Source: CAD feature listing. Evaluate the final solid. Frame: model axes, mm. Give positions to 0.01 mm unless a question says otherwise; leave off trailing zeros. Loops run counter-clockwise (first coordinate to the right, second up) from the corner with the lowest first, then second, coordinate; pieces in that order, holes last. Notation, with made-up numbers: (-6, 28) -> (37, 28) arc R18 cw to (37, 63) -> close; hole circle Ø5 at (24.25, 20). An arc over 180 degrees is marked (long way). Answer as a JSON object with one key per item and string values. Group by question number.
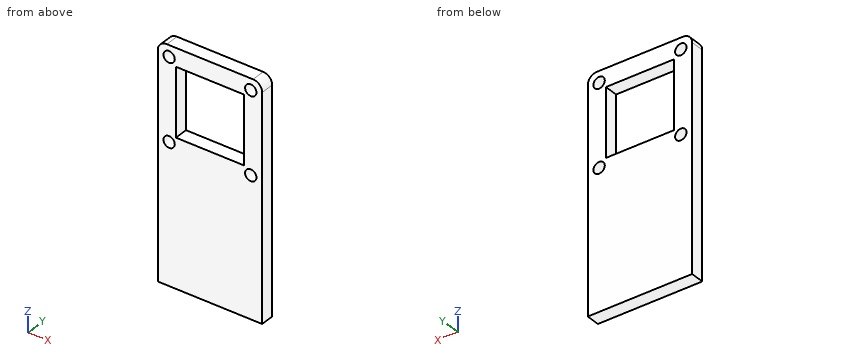
from build123d import *

# Parameters (mm, degrees)
F0_R     = 2.5
F0_W     = 30
F0_H     = 30
F1_DEPTH = 6


with BuildPart() as f1:
    # F0 (on Front) → F1 (new body)
    with BuildSketch(Plane.XZ):
        with BuildLine():
            ThreePointArc((23, 47), (21.828427, 49.828427), (19, 51))
            Line((19, 51), (-19, 51))
            ThreePointArc((-19, 51), (-21.828427, 49.828427), (-23, 47))
            Line((-23, 47), (-23, -51))
            Line((-23, -51), (23, -51))
            Line((23, -51), (23, 47))
        make_face()
        with Locations((-18, 10)):
            Circle(F0_R, mode=Mode.SUBTRACT)
        with Locations((-18, 46)):
            Circle(F0_R, mode=Mode.SUBTRACT)
        with Locations((18, 10)):
            Circle(F0_R, mode=Mode.SUBTRACT)
        with Locations((0, 28)):
            Rectangle(F0_W, F0_H, mode=Mode.SUBTRACT)
        with Locations((18, 46)):
            Circle(F0_R, mode=Mode.SUBTRACT)
    extrude(amount=F1_DEPTH)


solid = f1.part
(1) First-contact query: pin 1 (4 mm diameter, centred on x = -18, z = 10, fed in from -Y). Flat tip, straight axial feed; report the tip coordinate or a pass-through.
(2) Section query C-C on z = 10. Return the cut outline in (x, y), plus the area to 3 significant figures.
(3) Section query B-B on y = -3.05. Return the cut outline in (x, z), plus the area to 3 significant figures.
(4) Section query A-A on x = -7. Return the cut outline in (y, z).
(5) Section query D-D on x = -18. Return the cut outline in (y, z), plus the area to 3 significant figures.
(6) Material intervals for line 1 (Z direction, x = -18, y = -1.25); line 2 (X direction, y = -2, z = 30.5); line 3 (Z direction, x = 17, y = -1.85), sorted ascending. Write a range as from..to.
Result:
{
 "1": {"pin 1": "through"},
 "2": {"outline": "(-23, -6) -> (-20.5, -6) -> (-20.5, 0) -> (-23, 0) -> close; (-15.5, -6) -> (15.5, -6) -> (15.5, 0) -> (-15.5, 0) -> close; (20.5, -6) -> (23, -6) -> (23, 0) -> (20.5, 0) -> close", "area": "216 mm²"},
 "3": {"outline": "(-23, -51) -> (23, -51) -> (23, 47) arc R4 ccw to (19, 51) -> (-19, 51) arc R4 ccw to (-23, 47) -> close; hole circle Ø5 at (-18, 10); hole circle Ø5 at (-18, 46); hole (-15, 13) -> (15, 13) -> (15, 43) -> (-15, 43) -> close; hole circle Ø5 at (18, 10); hole circle Ø5 at (18, 46)", "area": "3,710 mm²"},
 "4": {"outline": "(-6, -51) -> (0, -51) -> (0, 13) -> (-6, 13) -> close; (-6, 43) -> (0, 43) -> (0, 51) -> (-6, 51) -> close"},
 "5": {"outline": "(-6, -51) -> (0, -51) -> (0, 7.5) -> (-6, 7.5) -> close; (-6, 12.5) -> (0, 12.5) -> (0, 43.5) -> (-6, 43.5) -> close; (-6, 48.5) -> (0, 48.5) -> (0, 51) -> (-6, 51) -> close", "area": "552 mm²"},
 "6": {"line 1": "-51..7.5, 12.5..43.5, 48.5..51", "line 2": "-23..-15, 15..23", "line 3": "-51..7.71, 12.29..43.71, 48.29..51"}
}
